Study the drawing (mm; zero at the part's minimum x, y, z) and answer. A direction names the side the tool comes from. Coordinates: 2 decimals unless noted, no trailing zeros. Write each loop counter-clockwise with the first axis right and the second up, starting at its lowest first coordinate (ties: lowest second). Pieces come first, ordered by that corner, then holes. Notation, with made-up numbers: M 20,-40 L 47,-40 A13 ccw 47,-18 Z; hole C 22.25,10.25 d10. An arc over 180 degrees is marked long. Answer as CSV lines item,"result". Start each with the question number.
(1) A cutting plane is placed at C-C on z = 2. Give the vertices of the cut face in (x, y) (3 decimals), then the cut area to 3 significant figures.
(2) A cutting plane is placed at A-A on z = 9. Give the vertices of the cut face in (x, y).
(3) For the marked faces 1 and 2, determine the directions among +Z, -Z, +X, -X, +Y, -Y from which every point of the face is accessible in a straight line to the end or side of a thin tool.
(4) Find the intervals of material crossed by L1, parallel to Y at x = 1.55, z = 9; L2, parallel to Y at x = 2.75, z = 15.5; L3, parallel to X at y = 9, z = 7.5, in increasing order. Write a range as [from, to].
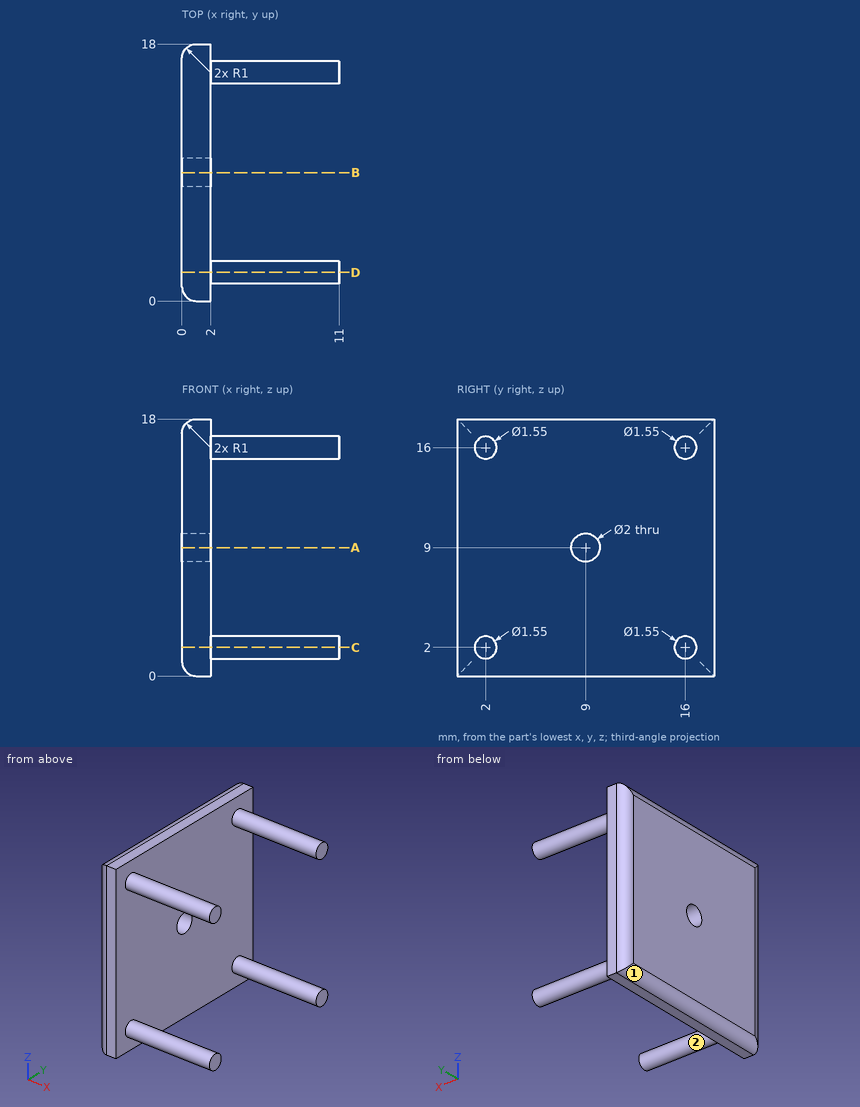
Here are the results:
1,outline,"M 0,1 A1 ccw 1,0 L 2,0 L 2,1.225 L 11,1.225 L 11,2.775 L 2,2.775 L 2,15.225 L 11,15.225 L 11,16.775 L 2,16.775 L 2,18 L 1,18 A1 ccw 0,17 Z"
1,area,"63.5 mm^2"
2,outline,"M 0,1 A1 ccw 1,0 L 2,0 L 2,8 L 0,8 Z; M 0,10 L 2,10 L 2,18 L 1,18 A1 ccw 0,17 Z"
3,face 1,"-Z, -X, +Y, -Y"
3,face 2,"+X"
4,L1,"y = [0, 8], [10, 18]"
4,L2,"y = [1.41, 2.59], [15.41, 16.59]"
4,L3,"x = [0, 2]"
